Verification items for the finished model (mm, model axes). A direction names the side the tool comes from. Round coordinates to 2 decimals unless told otherwise and drop trailing zeros. Order: outer loops, then holes, each group sorted by start corner. A loop starts at its lowest first (then second) coordinate and runs counter-clockwise, first axis right, second up. Notation, with made-up numbers: M 22,53.25 L 26,53.25 A26 cw 26,90.25 Z; hole C 9,-23 d6. An arc over 180 degrees is marked long. Return JSON: item names as keys, results as strings. Group by question number.
from build123d import *

# Parameters (mm, degrees)
ESBO_O1_W                = 118
ESBO_O1_H                = 88
RESSALTO_EXTRUS_O1_DEPTH = 2
FILETE1_R                = 10
FILETE2_R                = 10
ESBO_O2_W                = 42.31
ESBO_O2_H                = 42.4
CORTE_EXTRUS_O2_DEPTH    = 2
FILETE3_R                = 10
ESBO_O5_W                = 5
ESBO_O5_H                = 50
RESSALTO_EXTRUS_O3_DEPTH = 2
RESSALTO_EXTRUS_O4_START = -10
ESBO_O6_W                = 5
ESBO_O6_H                = 50
RESSALTO_EXTRUS_O4_DEPTH = 2


with BuildPart() as part:
    # Esboço1 → Ressalto-extrusão1 (new body)
    with BuildSketch(Plane(origin=(0, 0, 0), x_dir=(1, 0, 0), z_dir=(0, 1, 0))):
        Rectangle(ESBO_O1_W, ESBO_O1_H)
    extrude(amount=RESSALTO_EXTRUS_O1_DEPTH)

    # Filete1
    filete1_edges = [part.edges().sort_by_distance(p)[0] for p in [
        (59, 1, -44),
    ]]
    fillet(filete1_edges, radius=FILETE1_R)

    # Filete2
    filete2_edges = [part.edges().sort_by_distance(p)[0] for p in [
        (59, 1, 44),
        (-59, 1, 44),
        (-59, 1, -44),
    ]]
    fillet(filete2_edges, radius=FILETE2_R)

    # Esboço2 → Corte-extrusão2 (cut)
    with BuildSketch(Plane(origin=(0, 0, 0), x_dir=(1, 0, 0), z_dir=(0, 1, 0))):
        with Locations((1.985, 14.29)):
            Rectangle(ESBO_O2_W, ESBO_O2_H)
    extrude(amount=CORTE_EXTRUS_O2_DEPTH, mode=Mode.SUBTRACT)

    # Filete3
    filete3_edges = [part.edges().sort_by_distance(p)[0] for p in [
        (-19.17, 1, -35.49),
        (-19.17, 1, 6.91),
        (23.14, 1, 6.91),
        (23.14, 1, -35.49),
    ]]
    fillet(filete3_edges, radius=FILETE3_R)

    # Esboço5 → Ressalto-extrusão3 (add)
    with BuildSketch(Plane(origin=(59, 0, 0), x_dir=(0, 0, -1), z_dir=(1, 0, 0))):
        with Locations((-23.3, -22.870840319)):
            Rectangle(ESBO_O5_W, ESBO_O5_H)
        with Locations((23.3, -22.870840319)):
            Rectangle(ESBO_O5_W, ESBO_O5_H)
    extrude(amount=RESSALTO_EXTRUS_O3_DEPTH)

    # Esboço6 → Ressalto-extrusão4 (add)
    with BuildSketch(Plane.ZY.offset(69).offset(RESSALTO_EXTRUS_O4_START)):
        with Locations((-23.3, -22.870840319)):
            Rectangle(ESBO_O6_W, ESBO_O6_H)
        with Locations((23.3, -22.870840319)):
            Rectangle(ESBO_O6_W, ESBO_O6_H)
    extrude(amount=RESSALTO_EXTRUS_O4_DEPTH)


solid = part.part
1. Go/stop test with flat-tipped pins: pin 1 (1 mm diameter, centred on y = 1, z = -11.5, fed in from +X); pin 2 (10 mm diameter, centred on x = -6, z = -3, fed in from -Y); pin 3 (2 mm diameter, centred on x = -60.5, y = -18.5, fed in from -Z); pin 4 (1 mm diameter, centred on x = 60, y = -31.5, fed in from +Z). Record where each tip stops, or that it passes through.
2. Draft check along Z on faces 1 (the face through (20.29, 1.01, -32.48)), 2 (the face through (56.15, 1.01, 40.99)), 3 (the face through (-55.99, 1.01, -41.15)), 4 (the face through (-1, 0, 9)). Enter one of: +Z half, -Z half, draft (parallel to the pull), parting line (faces both ways), or undercut.
3. Thickness scan on line 1 along X through (y, z) = (-29, -22); line 2 along Y through (x, z) = (-47.5, 38.5). Record the ranges inside material, lowest first. Write a range as from..to.
4. Cross-section at B-B (y = -36). Enter the section's corners in (x, z).
5. Access from +Z, -Z, +X, -X, +Y, -Y to the whole of each face (thin tool, end or side, straight path). Record for faces 5 (the face through (20.13, 1.01, 4.06)), 6 (the face through (-61, -23, 23)), 7 (the face through (59, -24, 23)).
6. Cross-section at D-D (z = 18). Enter the section's corners in (x, y).
7. Cross-section at A-A (z = -6). Enter the section's corners in (x, y), plus the area to 3 significant figures.
8. Cross-section at C-C (x = 8.5). Enter the section's corners in (y, z), plus the area to 3 significant figures.
Computed:
{
 "1": {"pin 1": "stops at x = 59", "pin 2": "passes through", "pin 3": "stops at z = -25.8", "pin 4": "stops at z = 25.8"},
 "2": {"face 1": "undercut", "face 2": "+Z half", "face 3": "-Z half", "face 4": "draft"},
 "3": {"line 1": "x = -61..-59, 59..61", "line 2": "y = 0..2"},
 "4": {"outline": "M -61,-25.8 L -59,-25.8 L -59,-20.8 L -61,-20.8 Z; M -61,20.8 L -59,20.8 L -59,25.8 L -61,25.8 Z; M 59,-25.8 L 61,-25.8 L 61,-20.8 L 59,-20.8 Z; M 59,20.8 L 61,20.8 L 61,25.8 L 59,25.8 Z"},
 "5": {"face 5": "+Y, -Y", "face 6": "+Z, -Z, -X, +Y, -Y", "face 7": "+Z, -Z, -Y"},
 "6": {"outline": "M -59,0 L 59,0 L 59,2 L -59,2 Z"},
 "7": {"outline": "M -59,0 L -19.17,0 L -19.17,2 L -59,2 Z; M 23.14,0 L 59,0 L 59,2 L 23.14,2 Z", "area": "151 mm²"},
 "8": {"outline": "M 0,-44 L 2,-44 L 2,-35.49 L 0,-35.49 Z; M 0,6.91 L 2,6.91 L 2,44 L 0,44 Z", "area": "91.2 mm²"}
}
